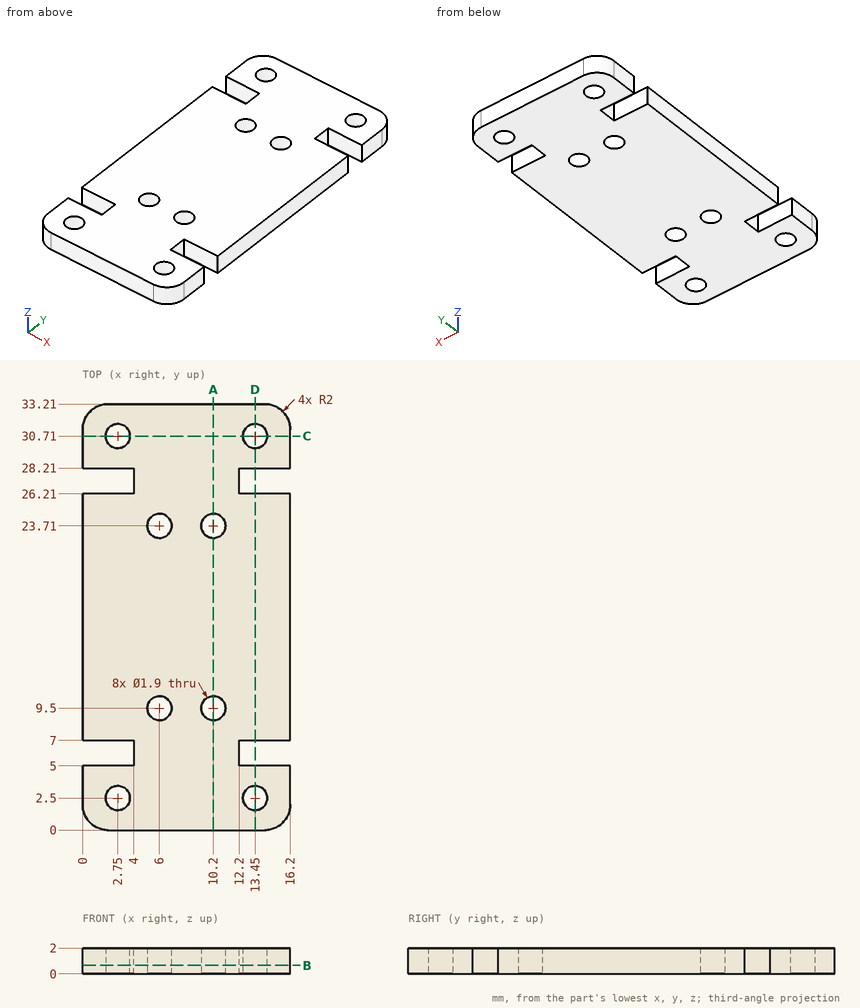
Design review of the part shown in the three views and the two pictorial views. Dimensions are in mm from the part's minimum x, y and z. Coordinates: 2 decimals unless noted, no trailing zeros. Loops run counter-clockwise (first coordinate to the right, second up) from the corner with the lowest first, then second, coordinate; pieces in that order, holes last. Notation, with made-up numbers: (-20.75, -20) - (-16.75, -20) arc R17 cw to (-16.75, 12) - close; hole circle Ø6 at (71.5, 9). An arc over 180 degrees is marked (long way). Use a Markdown table: item, result. Add a question column.
Item 1: We need section B-B (z = 0.65). Give the number of separate pieces and of enclosed holes in the cut face, and give its area (3 significant figures).
Item 2: We need section C-C (y = 30.71). Give the boundary of the cut face in (x, z), and give its area (3 significant figures).
Item 3: We need section A-A (x = 10.2). Give the boundary of the cut face in (y, z).
Item 4: Insertion check: pin 1 Ø1 at (y, z) = (27.5, 1) entering from -X; pin 2 Ø0.6 at (x, z) = (1.5, 1.5) entering from +Y. Each pin has a flat end and moves straight along its axis. Give the tip position at first contact, or say it passes through.
Item 5: For line 1 (X direction, y = 9.5, z = 1.4); line 2 (Y direction, x = 6, z = 1); line 3 (Y direction, x = 2.75, z = 0.9), list the stretches that pass through material, from the lowest coordinate up.
Item 6: We need section D-D (x = 13.45). Give the boundary of the cut face in (y, z), and give its area (3 significant figures).
Results list:
| question | item | result |
|---|---|---|
| 1 | separate pieces | 1 |
| 1 | enclosed holes | 8 |
| 1 | area | 480 mm^2 |
| 2 | outline | (0, 0) - (1.8, 0) - (1.8, 2) - (0, 2) - close; (3.7, 0) - (12.5, 0) - (12.5, 2) - (3.7, 2) - close; (14.4, 0) - (16.2, 0) - (16.2, 2) - (14.4, 2) - close |
| 2 | area | 24.8 mm^2 |
| 3 | outline | (0, 0) - (8.55, 0) - (8.55, 2) - (0, 2) - close; (10.45, 0) - (22.76, 0) - (22.76, 2) - (10.45, 2) - close; (24.66, 0) - (33.21, 0) - (33.21, 2) - (24.66, 2) - close |
| 4 | pin 1 | stops at x = 4 |
| 4 | pin 2 | stops at y = 33.2 |
| 5 | line 1 | x = 0 to 5.05, 6.95 to 9.25, 11.15 to 16.2 |
| 5 | line 2 | y = 0 to 8.55, 10.45 to 22.76, 24.66 to 33.21 |
| 5 | line 3 | y = 0 to 1.55, 3.45 to 5, 7 to 26.21, 28.21 to 29.76, 31.66 to 33.21 |
| 6 | outline | (0, 0) - (1.55, 0) - (1.55, 2) - (0, 2) - close; (3.45, 0) - (5, 0) - (5, 2) - (3.45, 2) - close; (7, 0) - (26.21, 0) - (26.21, 2) - (7, 2) - close; (28.21, 0) - (29.76, 0) - (29.76, 2) - (28.21, 2) - close; (31.66, 0) - (33.21, 0) - (33.21, 2) - (31.66, 2) - close |
| 6 | area | 50.8 mm^2 |
